Read the model definition and answer for the solid it produces. Units are mm, in the model's axes. Face numbers are marked on the shaded views. A direction names the side the tool comes from. Give positions to 0.01 mm unless a question says otherwise; leave off trailing zeros. Loops run counter-clockwise (first coordinate to the right, second up) from the corner with the lowest first, then second, coordinate; pieces in that order, holes last. Notation, with made-up numbers: (-20.75, 22) -> (-11.75, 22) arc R10 cw to (-11.75, 26) -> close; hole circle Ø2 at (67.25, -0.75). An arc over 180 degrees is marked (long way). Write each question's results on one line, items separated by ' | '. Start each with the question number.
Item 1: Section D-D on x = 0 is taken. Write down the section's boundary in (y, z), and give its area (3 significant figures).
Item 2: Section C-C on y = -7 is taken. Write down the section's boundary in (x, z), and give its area (3 significant figures).
Item 3: Section A-A on x = 11.75 is taken. Write down the section's boundary in (y, z), and give its area (3 significant figures).
Item 4: Each of these flat-tipped pins is pushed along its axis until it touches: P1, Ø2.5, axis at x = -23.5, z = 0, coming from the +Y side; P2, Ø1.2, axis at y = 6, z = -13, coming from the -X side; P3, Ø14.5, axis at x = 1.5, z = 0.5, coming from the -Y side; P4, Ø11, axis at y = -6.5, z = 3, coming from the +X side. Where does it stop, or does it pass through?
Item 5: Which of the six approach directions +Z, -Z, +X, -X, +Y, -Y give full straight-line access (tool end or side, diameter ignored) to the marked faces 4, 5, 6, 7 and 8?
Item 6: Find the intervals of material crossed by line 1 (Z direction, x = 12.5, y = 3.25); line 2 (Y direction, x = -15, z = 9); line 3 (Z direction, x = 12.25, y = -7), in increasing order.
Item 7: Section B-B on y = -2 is taken. Write down the section's boundary in (x, z).
Item 8: Determine the mould class of the marked faces 1, 2 and 3 for opening direction Z: +Z half, -Z half, draft (parallel to the pull), parting line (faces both ways), or undercut.
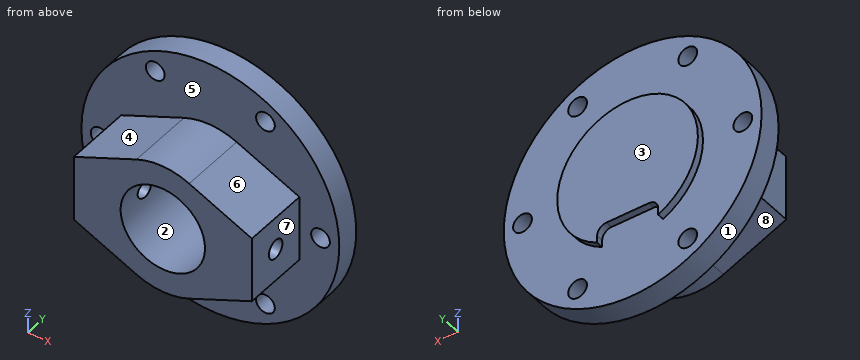
Autodesk Inventor part; units mm, degrees
ref_plane "YZ Plane" through (0, 0, 0) normal (1, 0, 0) x (0, 1, 0)
ref_plane "XZ Plane" through (0, 0, 0) normal (0, 1, 0) x (-1, 0, 0)
ref_plane "XY Plane" through (0, 0, 0) normal (0, 0, 1) x (1, 0, 0)
sketch "Skizze1" plane through (0, 0, 0) normal (0, 1, 0) x (-1, 0, 0)
  circle A0 centre (0, 0) radius 27.5
  dimension "d0" = 55
extrude "Extrusion1" add sketch "Skizze1" along normal blind 5
sketch "Skizze2" plane through (0, 5, 0) normal (0, 1, 0) x (1, 0, 0)
  circle A0 centre (0, 0) radius 15
  dimension "d4" = 30
extrude "Extrusion2" add sketch "Skizze2" along normal blind 1.5
sketch "Skizze3" plane through (0, 6.5, 0) normal (0, 1, 0) x (1, 0, 0)
  circle A0 centre (0, 0) radius 15
  line L0 (-6.5, 13.5185) -> (-6.5, 12)
  line L1 (-4.5, 10) -> (4.5, 10)
  line L2 (6.5, 12) -> (6.5, 13.5185)
  line L3 (0, -15) -> (0, 15) construction
  arc A1 (-6.5, 12) -> (-4.5, 10) centre (-4.5, 12) ccw
  arc A2 (4.5, 10) -> (6.5, 12) centre (4.5, 12) ccw
  point P0 (-6.5, 10)
  point P1 (6.5, 10)
  dimension "d7" = 13
  dimension "d8" = 10
  dimension "d9" = 2
extrude "Extrusion3" cut sketch "Skizze3" against normal blind 1.5 contours L2 A2 L1 A1 L0 A0 picked at (0, 11.6667)
sketch "Skizze4" plane through (0, 5, 0) normal (0, 1, 0) x (1, 0, 0)
  circle A0 centre (0, 0) radius 23.5 construction
  point P0 (-23.5, 0)
  dimension "d12" = 47
hole "Bohrung1" at (-23.5, 5, 0) direction (0, -1, 0) diameter 4 end through all
pattern_circular "Runde Anordnung1" count 6 over 360 about axis through (0, 0, 0) along (0, 1, 0) of "Bohrung1"
sketch "Skizze5" plane through (0, 0, 0) normal (0, -1, 0) x (1, 0, 0)
  line L0 (-19, -7) -> (-19, 7)
  line L1 (-19, 7) -> (-5.6144, 12.8489)
  line L2 (-19, -7) -> (-5.6144, -12.8489)
  line L3 (5.6144, -12.8489) -> (19, -7)
  line L4 (19, -7) -> (19, 7)
  line L5 (19, 7) -> (5.6144, 12.8489)
  line L6 (0, -28.3232) -> (0, 28.3232) construction
  arc A0 (-5.6144, -12.8489) -> (5.6144, -12.8489) centre (0, 0) ccw
  arc A1 (5.6144, 12.8489) -> (-5.6144, 12.8489) centre (0, 0) ccw
  point P0 (-19, 0)
  point P1 (19, 0)
  dimension "d27" = 14
  dimension "d28" = 14
  dimension "d29" = 38
extrude "Extrusion4" add sketch "Skizze5" along normal blind 14
sketch "Skizze6" plane through (0, -14, 0) normal (0, -1, 0) x (1, 0, 0)
  circle A0 centre (0, 0) radius 9
  dimension "d32" = 18
extrude "Extrusion5" cut sketch "Skizze6" against normal blind 15.5
thread "Gewinde1"
sketch "Skizze7" plane through (-19, 0, -7) normal (-1, 0, 0) x (0, 0, 1)
  line L0 (-5.8489, 0) -> (-5.8489, -14)
  line L1 (0, 0) -> (14, 0)
  point P0 (7, 0)
  point P1 (7, -7)
  point P2 (-5.8489, -7)
  point P3 (7, 0)
hole "Bohrung2" at (-19, -7, 0) direction (1, 0, 0) diameter 4 depth 10 tip angle 118
mirror "Mirror1" about plane through (0, 0, 0) normal (1, 0, 0) of "Bohrung2"
properties part number "109" material "Gold"
Findings:
1) outline: (-14, -14.02) -> (0, -14.02) -> (0, -27.5) -> (5, -27.5) -> (5, -10) -> (6.5, -10) -> (6.5, 15) -> (5, 15) -> (5, 27.5) -> (0, 27.5) -> (0, 14.02) -> (-14, 14.02) -> (-14, 9) -> (1.5, 9) -> (1.5, -9) -> (-14, -9) -> close | area: 426 mm2
2) outline: (-19, -7) -> (-5.61, -12.85) arc R14.02 ccw to (5.61, -12.85) -> (19, -7) -> (19, -2) -> (9, -2) -> (8.83, -1.72) arc R9 cw to (-8.83, -1.72) -> (-9, -2) -> (-19, -2) -> close; (-19, 2) -> (-9, 2) -> (-8.83, 1.72) arc R9 cw to (8.83, 1.72) -> (9, 2) -> (19, 2) -> (19, 7) -> (5.61, 12.85) arc R14.02 ccw to (-5.61, 12.85) -> (-19, 7) -> close | area: 503 mm2
3) outline: (-14, -10.17) -> (0, -10.17) -> (0, -18.35) -> (5, -18.35) -> (5, -9.32) -> (6.5, -9.32) -> (6.5, 9.32) -> (5, 9.32) -> (5, 18.35) -> (0, 18.35) -> (0, 10.17) -> (-14, 10.17) -> close; (0, -24.86) -> (5, -24.86) -> (5, -22.35) -> (0, -22.35) -> close; (0, 22.35) -> (5, 22.35) -> (5, 24.86) -> (0, 24.86) -> close; hole circle Ø4 at (-7, 0) | area: 509 mm2
4) P1: through | P2: x = -8.44 | P3: y = 1.5 | P4: x = 19
5) face 4: +Z, -X, -Y | face 5: -Y | face 6: +Z, +X, -Y | face 7: +Z, -Z, +X, -Y | face 8: -Z, -X, -Y
6) line 1: -24.49 to -22.21, -18.5 to 18.5, 22.21 to 24.49 | line 2: 0 to 5 | line 3: -9.95 to -2, 2 to 9.95
7) outline: (-19, -7) -> (-5.61, -12.85) arc R14.02 ccw to (5.61, -12.85) -> (19, -7) -> (19, 7) -> (5.61, 12.85) arc R14.02 ccw to (-5.61, 12.85) -> (-19, 7) -> close; hole circle Ø18 at (0, 0)
8) face 1: parting line | face 2: undercut | face 3: draft
